The model under review builds one solid part; all positions refer to its coordinate system, in mm. A direction names the side the tool comes from. Give positions to 0.01 mm unless a question says otherwise; leave off trailing zeros. Order: outer loops, then holes, each group sorted by start corner. A loop starts at its lowest first (then second) coordinate and runs counter-clockwise, first axis right, second up. Notation, with made-up numbers: (46, 63.25) - (57, 63.25) arc R30 ccw to (57, 101.25) - close; hole circle Ø11 at (-8, 55.5). An arc over 180 degrees is marked (long way). Put each result on its own line as item: value.
Autodesk Inventor part; units mm, degrees
ref_plane "YZ Plane" through (0, 0, 0) normal (1, 0, 0) x (0, 1, 0)
ref_plane "XZ Plane" through (0, 0, 0) normal (0, 1, 0) x (-1, 0, 0)
ref_plane "XY Plane" through (0, 0, 0) normal (0, 0, 1) x (1, 0, 0)
sketch "Эскиз1" plane through (0, 0, 0) normal (0, 1, 0) x (-1, 0, 0)
  circle A0 centre (-44.87, 82.9015) radius 1.5
  line L0 (-31, 99.2724) -> (-31, 78.7724)
  line L1 (-31, 78.7724) -> (31, 78.7724)
  circle A1 centre (-42.22, 16) radius 1.5
  circle A2 centre (-16, 42.22) radius 1.5
  circle A3 centre (16, 42.22) radius 1.5
  circle A4 centre (31, 72.43) radius 1.5
  circle A5 centre (16, 72.43) radius 1.5
  circle A6 centre (-16, 72.43) radius 1.5
  arc A7 (-31, 99.2724) -> (-99.2724, 31) centre (0, 0) ccw
  circle A8 centre (-74.5664, 57.67) radius 1.5
  circle A9 centre (-82.9015, 44.87) radius 1.5
  circle A10 centre (-72.43, -16) radius 1.5
  circle A11 centre (-72.43, 16) radius 1.5
  line L2 (-78.7724, 31) -> (-78.7724, -31)
  line L3 (-99.2724, 31) -> (-78.7724, 31)
  line L4 (31, 78.7724) -> (31, 99.2724)
  arc A12 (34.57, 98.0863) -> (98.0863, 34.57) centre (109.0212, 109.0212) ccw
  circle A13 centre (72.43, 31) radius 1.5
  line L5 (99.2724, 31) -> (78.7724, 31)
  circle A14 centre (72.43, 16) radius 1.5
  arc A15 (34.57, 98.0863) -> (31, 99.2724) centre (0, 0) ccw
  arc A16 (99.2724, 31) -> (98.0863, 34.57) centre (0, 0) ccw
  arc A17 (98.0863, 34.57) -> (34.57, 98.0863) centre (0, 0) ccw
  circle A18 centre (42.22, 16) radius 1.5
  circle A19 centre (82.9015, -44.87) radius 1.5
  line L6 (78.7724, -31) -> (99.2724, -31)
  arc A20 (31, -99.2724) -> (99.2724, -31) centre (0, 0) ccw
  circle A21 centre (16, -72.43) radius 1.5
  line L7 (31, -78.7724) -> (31, -99.2724)
  circle A22 centre (44.87, -82.9015) radius 1.5
  circle A23 centre (57.67, -74.5664) radius 1.5
  circle A24 centre (-57.67, 74.5664) radius 1.5
  circle A25 centre (-42.22, -16) radius 1.5
  circle A26 centre (42.22, -16) radius 1.5
  circle A27 centre (-72.43, -31) radius 1.5
  line L8 (-73.5391, 73.5391) -> (73.5391, -73.5391) construction
  line L9 (78.7724, 31) -> (78.7724, -31)
  circle A28 centre (72.43, -16) radius 1.5
  circle A29 centre (-16, -42.22) radius 1.5
  circle A30 centre (16, -42.22) radius 1.5
  circle A31 centre (74.5664, -57.67) radius 1.5
  line L10 (-31, -78.7724) -> (31, -78.7724)
  circle A32 centre (-16, -72.43) radius 1.5
  circle A33 centre (-31, -72.43) radius 1.5
  line L11 (-31, -99.2724) -> (-31, -78.7724)
  arc A34 (-34.57, -98.0863) -> (-31, -99.2724) centre (0, 0) ccw
  line L12 (-78.7724, -31) -> (-99.2724, -31)
  arc A35 (-99.2724, -31) -> (-98.0863, -34.57) centre (0, 0) ccw
  arc A36 (-98.0863, -34.57) -> (-34.57, -98.0863) centre (0, 0) ccw
  arc A37 (-34.57, -98.0863) -> (-98.0863, -34.57) centre (-109.0212, -109.0212) ccw
sketch "Эскиз2" plane through (0, 0, 0) normal (0, 1, 0) x (-1, 0, 0)
  arc A0 (34.57, 98.0863) -> (98.0863, 34.57) centre (109.0212, 109.0212) ccw
  arc A1 (99.2724, 31) -> (98.0863, 34.57) centre (0, 0) ccw
  arc A2 (34.57, 98.0863) -> (31, 99.2724) centre (0, 0) ccw
  line L0 (31, 78.7724) -> (31, 99.2724)
  circle A3 centre (31, 72.43) radius 1.5
  circle A4 centre (72.43, 31) radius 1.5
  circle A5 centre (31, 72.43) radius 4.5
  circle A6 centre (72.43, 31) radius 4.5
  line L1 (27.818, 69.248) -> (69.248, 27.818)
  line L2 (26.5, 78.7724) -> (26.5, 72.43)
  line L3 (78.7724, 31) -> (78.7724, -31)
  line L4 (78.7724, 26.5) -> (72.43, 26.5)
  line L5 (99.2724, 31) -> (78.7724, 31)
  line L6 (26.5, 78.7724) -> (31, 78.7724)
  dimension "d0" = 9
  dimension "d1" = 9
extrude "Выдавливание1" add sketch "Эскиз2" along normal blind 32
ref_plane "РабПлоскость1" through (0, 25.3, 0) normal (0, 1, 0) x (1, 0, 0)
sketch "Эскиз3" plane through (0, 25.3, 0) normal (0, 1, 0) x (1, 0, 0)
  circle A0 centre (-72.43, -31) radius 1.5
  circle A1 centre (-31, -72.43) radius 1.5
  point P0 (0, 0)
extrude "Выдавливание2" add sketch "Эскиз3" against normal blind 20.6
sketch "Эскиз4" plane through (-31, 0, 78.7724) normal (0, 0, 1) x (1, 0, 0)
  line L0 (0, 1) -> (0, 32)
  line L1 (0, 32) -> (-3.57, 32)
  line L2 (0, 0) -> (0, 32)
  arc A0 (0, 32) -> (0, 0) centre (72.5929, 16) ccw
  point P0 (31, 0)
extrude "Выдавливание3" cut sketch "Эскиз4" along normal through all
ref_plane "РабПлоскость2" through (-48.533, 0, 48.533) normal (0.7071, 0, 0.7071) x (0, 1, 0)
mirror "Зеркальное отражение1" about plane through (-48.533, 0, 48.533) normal (0.7071, 0, 0.7071) of "Выдавливание3"
sketch "Эскиз6" plane through (0, 0, 0) normal (0, 1, 0) x (1, 0, 0)
  circle A0 centre (124.1994, 64.0459) radius 3
  circle A1 centre (-31, -72.43) radius 1.5
  circle A2 centre (-72.43, -31) radius 1.5
  line L0 (-72.43, -31) -> (-31, -72.43)
  line L1 (-31, -72.43) -> (-36.2927, -77.7227)
  circle A3 centre (-36.2927, -77.7227) radius 2
  line L2 (164.6688, 164.6688) -> (-154.6363, -154.6363)
  circle A4 centre (-77.7227, -36.2927) radius 2
  point P0 (0, 0)
  point P1 (129.0863, 44.2024)
  dimension "d12" = 6
  dimension "d13" = 7.485
  dimension "d14" = 4
extrude "Выдавливание5" cut sketch "Эскиз6" along normal blind 7 contours A3 | A4
ref_plane "РабПлоскость4" through (0, 12.8, 0) normal (0, -1, 0) x (1, 0, 0)
sketch "Эскиз9" plane through (0, 12.8, 0) normal (0, -1, 0) x (1, 0, 0)
  line L0 (-83.2724, 34) -> (-96.2724, 34)
  line L1 (-96.2724, 34) -> (-96.2724, 31)
  line L2 (-96.2724, 31) -> (-83.2724, 31)
  line L3 (-83.2724, 31) -> (-83.2724, 34)
  line L4 (-99.2724, 31) -> (-78.7724, 31)
  point P0 (0, 0)
  point P1 (0, 0)
  dimension "d23" = 3
  dimension "d24" = 13
  dimension "d43" = 3
extrude "Выдавливание6" cut sketch "Эскиз9" along normal mid plane 5.15
sketch "Эскиз10" plane through (-48.533, 0, 48.533) normal (0.7071, 0, 0.7071) x (0, 1, 0)
  line L0 (15.375, 14.288) -> (10.225, 14.288)
  line L1 (12.8, 14.288) -> (12.8, 27.3139)
  circle A0 centre (12.8, 19.5665) radius 1.5
  line L2 (0, 5.8027) -> (32, 5.8027)
  point P0 (0, -68.6361)
  dimension "d29" = 3
  dimension "d31" = 13.7638
extrude "Выдавливание7" cut sketch "Эскиз10" along normal mid plane 100
hole "Отверстие1" at (-72.43, 0, 31) at (-31, 0, 72.43) direction (0, 1, 0) diameter 4 depth 4.7
sketch "Эскиз11" plane through (0, 32, 0) normal (0, 1, 0) x (1, 0, 0)
  circle A0 centre (-72.43, -31) radius 1.5
  circle A1 centre (-31, -72.43) radius 1.5
  circle A2 centre (-72.43, -31) radius 2
  circle A3 centre (-31, -72.43) radius 2
  point P0 (0, 0)
extrude "Выдавливание8" cut sketch "Эскиз11" against normal up to surface (6.7 mm away) contours A0 | A1 | A2 | A3
equation "\"d1\" = d0"
properties part number "сфеср"
(1) The part is to be moulded in two halves that separate along Z. For faces 1 (the flat face through (-55, 32, 52)), 2 (the flat face through (-31, 25.3, 72)), 3 (the cylindrical face through (-98.554, 15.776, 33.212)), 4 (the flat face through (-31, 4.7, 72)), say which applies: pulls with the +Z half, pulls with the -Z half, needs draft (parallel to the pull), parting line crosses it, or undercut.
The answers:
face 1: needs draft
face 2: undercut
face 3: pulls with the +Z half
face 4: undercut
(2) Wall thickness on L1, parallel to Y at x = -93, z = 33.5 (3 decimals); L2, parallel to Z at x = -31, y = 30.75; L3, parallel to X at y = 27, z = 31: over which ranges is each line inside the solid? List them lowest first.
The answers:
L1: 0 to 10.225, 15.375 to 32
L2: 66.07 to 70.43, 74.43 to 78.77
L3: -78.77 to -74.43, -70.43 to -66.07
(3) For faces 5 (the flat face through (-78, 7, 36)), 6 (the flat face through (-78.772, 16, 30)), 7 (the cylindrical face through (-32.74, 15.77, 88.88)), list the 3-axis set-ups (+Z, -Z, +X, -X, +Y, -Y) from which the entire face can be reached by the end or side of a thin tool; tool diameter is ignored.
The answers:
face 5: -Y
face 6: -Z, -X
face 7: +Z, +X
(4) Take a section at A-A, the plane y = 27. Write out the cut boundary in (x, z).
The answers:
outline: (-98.98, 31.92) - (-78.77, 31.92) - (-78.77, 26.5) - (-72.43, 26.5) arc R4.5 ccw to (-69.25, 27.82) - (-27.82, 69.25) arc R4.5 ccw to (-26.5, 72.43) - (-26.5, 78.77) - (-31.92, 78.77) - (-31.92, 98.98) arc R104.03 ccw to (-34.57, 98.09) arc R75.25 cw to (-98.09, 34.57) arc R103.97 ccw to start; hole circle Ø4 at (-72.43, 31); hole circle Ø4 at (-31, 72.43)
(5) Clearance check with flat-ended pins moving along their axes: pin 1 Ø2 at (x, z) = (-36.5, 77.5) entering from -Y; pin 2 Ø12 at (x, y) = (-57.5, 15.5) entering from +Z; pin 3 Ø2 at (x, y) = (-82, 3.5) entering from +Z. State where each tip first meets the part, or that it passes through.
The answers:
pin 1: y = 7
pin 2: z = 60.5
pin 3: z = 39.18
(6) Take a section at D-D, the plane x = -44. Write out the cut boundary in (y, z).
The answers:
outline: (0, 53.07) - (32, 53.07) - (32, 71.14) - (0, 71.14) - close
(7) Take a section at C-C, the plane z = 46.5. Write out the cut boundary in (x, y), then the cut area to 3 significant figures.
The answers:
outline: (-67.14, 0) - (-50.57, 0) - (-50.57, 32) - (-67.14, 32) - close
area: 531 mm^2
(8) Take a section at B-B, the plane y = 8. Write out the cut boundary in (x, z), then the cut area to 3 significant figures.
The answers:
outline: (-98.85, 32.31) - (-78.77, 32.31) - (-78.77, 26.5) - (-72.43, 26.5) arc R4.5 ccw to (-69.25, 27.82) - (-27.82, 69.25) arc R4.5 ccw to (-26.5, 72.43) - (-26.5, 78.77) - (-32.31, 78.77) - (-32.31, 98.85) arc R104.03 ccw to (-34.57, 98.09) arc R75.25 cw to (-98.09, 34.57) arc R103.97 ccw to start
area: 1,000 mm^2
